Part model, mm, in its own coordinate system. Face numbers are marked on the shaded views. A direction names the side the tool comes from. Coordinates: 2 decimals unless noted, no trailing zeros. Loops run counter-clockwise (first coordinate to the right, second up) from the corner with the lowest first, then second, coordinate; pieces in that order, holes last. Notation, with made-up numbers: M 72,-26.5 L 88,-26.5 A19 cw 88,-9.5 Z; hole C -29,75.25 d3. An arc over 180 degrees is marked long. Use a Markdown table: item, result. Add a question column.
1) Band-saw the part on A-A (y = 19). State how many separate pieces and enclosed holes the cut face has, plus the area to 3 significant figures.
2) Wall check: probe 1 along Z at (x, y) = (1, 11.5); probe 2 along Z at (x, y) = (-2.5, 10.75); probe 3 along Y at (x, z) = (0, -39). Give the ranges that are in metal, low to high. Write a range as from..to.
3) Band-saw the part on D-D (z = -1.5). List the corners of the cut face in (x, y), plus the area to 3 significant figures.
4) Pull direction Z, two halves, no side cores. Call the marked faces 1, 2 and 3: released by +Z, released by -Z, zero draft, split by the parting line, or undercut.
5) Tool access for the marked faces 4 and 5: list every direction of +Z, -Z, +X, -X, +Y, -Y with a clear straight run to the whole face (end or side of a thin tool).
6) Band-saw the part on B-B (z = -31). List the corners of the cut face in (x, y), plus the area to 3 significant figures.
7) Pin check, flat tips, straight feed: pin 1 Ø4.5 at (y, z) = (7, 1) entering from +X; pin 2 Ø1.8 at (x, z) = (-13.5, 0.5) entering from +Y; pin 3 Ø3 at (x, y) = (0, 19) entering from +Z; pin 4 Ø3 at (x, z) = (0.5, -2.5) entering from +Y. Stop position of each tip, or through.
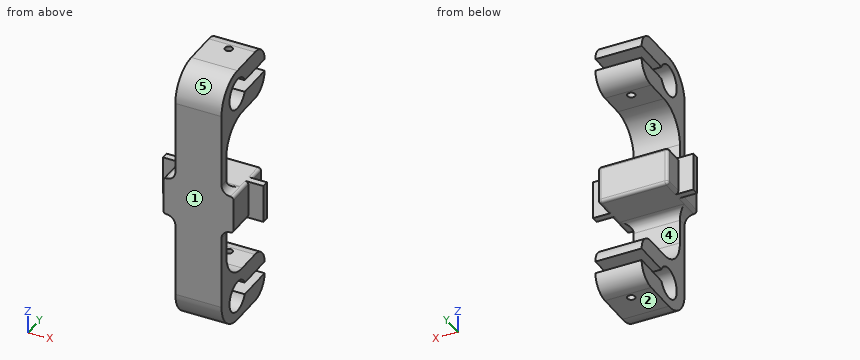
Autodesk Inventor part; units mm, degrees
ref_plane "YZ Plane" through (0, 0, 0) normal (1, 0, 0) x (0, 1, 0)
ref_plane "XZ Plane" through (0, 0, 0) normal (0, 1, 0) x (-1, 0, 0)
ref_plane "XY Plane" through (0, 0, 0) normal (0, 0, 1) x (1, 0, 0)
sketch "Schizzo1" plane through (0, 0, 0) normal (0, 1, 0) x (-1, 0, 0)
  line L0 (7.5, 43) -> (-7.5, 43)
  line L1 (-7.5, 43) -> (-7.5, -43)
  line L2 (-7.5, -43) -> (7.5, -43)
  line L3 (7.5, -43) -> (7.5, 43)
  line L4 (7.5, 43) -> (-7.5, -43) construction
  line L5 (-7.5, 43) -> (7.5, -43) construction
  point P0 (0, 0)
  dimension "d0" = 15
  dimension "d1" = 86
extrude "Estrusione1" add sketch "Schizzo1" along normal blind 3
sketch "Schizzo2" plane through (0, 3, 0) normal (0, 1, 0) x (1, 0, 0)
  line L0 (7.5, 43) -> (-7.5, 43)
  line L1 (-7.5, 43) -> (-7.5, 27)
  line L2 (-7.5, 27) -> (7.5, 27)
  line L3 (7.5, 27) -> (7.5, 43)
  line L4 (-7.5, 43) -> (-7.5, -43)
  line L5 (7.5, 43) -> (-7.5, 43)
  line L6 (-7.5, -43) -> (7.5, -43)
  line L7 (7.5, -43) -> (-7.5, -43)
  line L8 (-7.5, -43) -> (-7.5, -27)
  line L9 (-7.5, -27) -> (7.5, -27)
  line L10 (7.5, -27) -> (7.5, -43)
  point P0 (0, 0)
  dimension "d4" = 15
  dimension "d5" = 16
  dimension "d6" = 0
  dimension "d7" = 0
  dimension "d8" = 16
extrude "Estrusione2" add sketch "Schizzo2" along normal blind 24
sketch "Schizzo3" plane through (-7.5, 0, -43) normal (-1, 0, 0) x (0, 0, 1)
  line L0 (0, 0) -> (86, 0)
  line L1 (0, 0) -> (0, 27)
  line L2 (86, 0) -> (86, 27)
  circle A0 centre (8, 10) radius 5
  circle A1 centre (78, 10) radius 5
  point P0 (43, 0)
  dimension "d11" = 10
  dimension "d12" = 8
  dimension "d13" = 10
  dimension "d14" = 8
  dimension "d15" = 10
  dimension "d16" = 10
extrude "Estrusione3" cut sketch "Schizzo3" against normal blind 30
fillet "Raccordo1" radius 10 2 edges at (0, 3, -27) (0, 3, 27)
fillet "Raccordo2" radius 10 2 edges at (0, 0, -43) (0, 0, 43)
sketch "Schizzo4" plane through (0, 27, 0) normal (0, 1, 0) x (1, 0, 0)
  line L0 (7.5, 37) -> (-7.5, 37)
  line L1 (-7.5, 37) -> (-7.5, 33)
  line L2 (-7.5, 33) -> (7.5, 33)
  line L3 (7.5, 33) -> (7.5, 37)
  line L4 (7.5, 27) -> (7.5, 43)
  line L5 (7.5, 43) -> (-7.5, 43)
  line L6 (7.5, -33) -> (-7.5, -33)
  line L7 (-7.5, -33) -> (-7.5, -37)
  line L8 (-7.5, -37) -> (7.5, -37)
  line L9 (7.5, -37) -> (7.5, -33)
  line L10 (7.5, -43) -> (7.5, -27)
  line L11 (-7.5, -43) -> (7.5, -43)
  point P0 (0, 0)
  dimension "d21" = 15
  dimension "d22" = 4
  dimension "d23" = 0
  dimension "d24" = 6
  dimension "d25" = 15
  dimension "d26" = 4
  dimension "d27" = 0
  dimension "d28" = 6
extrude "Estrusione4" cut sketch "Schizzo4" against normal blind 15
sketch "Schizzo5" plane through (7.5, 27, -43) normal (0, 0, -1) x (-1, 0, 0)
  line L0 (0, 0) -> (15, 0)
  line L1 (15, -17) -> (15, 0)
  circle A0 centre (7.5, -8) radius 1.25
  point P0 (7.5, -27)
  dimension "d31" = 8
  dimension "d32" = 7.5
  dimension "d33" = 2.5
extrude "Estrusione5" cut sketch "Schizzo5" against normal blind 86
fillet "Raccordo3" radius 6 4 edges at (0, 27, 43) (0, 27, 27) (0, 27, -27) (0, 27, -43)
sketch "Schizzo6" plane through (0, 0, 0) normal (0, -1, 0) x (1, 0, 0)
  line L0 (-11.4, -6.2) -> (11.4, -6.2)
  line L1 (11.4, -6.2) -> (11.4, 6.2)
  line L2 (11.4, 6.2) -> (-11.4, 6.2)
  line L3 (-11.4, 6.2) -> (-11.4, -6.2)
  line L4 (-11.4, -6.2) -> (11.4, 6.2) construction
  line L5 (11.4, -6.2) -> (-11.4, 6.2) construction
  point P0 (0, 0)
  dimension "d37" = 22.8
  dimension "d38" = 12.4
extrude "Estrusione6" add sketch "Schizzo6" against normal blind 18
sketch "Schizzo7" plane through (11.4, 0, 6.2) normal (1, 0, 0) x (0, 0, -1)
  line L0 (0, 11.5) -> (12.4, 11.5)
  line L1 (12.4, 11.5) -> (12.4, 9.3)
  line L2 (12.4, 9.3) -> (0, 9.3)
  line L3 (0, 9.3) -> (0, 11.5)
  line L4 (0, 11.5) -> (12.4, 9.3) construction
  line L5 (12.4, 11.5) -> (0, 9.3) construction
  line L6 (12.4, 0) -> (0, 0)
  line L7 (12.4, 0) -> (12.4, 18)
  point P0 (6.2, 0)
  point P1 (6.2, 10.4)
  dimension "d41" = 12.4
  dimension "d42" = 2.2
  dimension "d43" = 9.3
  dimension "d44" = 0
extrude "Estrusione7" add sketch "Schizzo7" along normal blind 4.9
sketch "Schizzo8" plane through (-11.4, 0, -6.2) normal (-1, 0, 0) x (0, 0, 1)
  line L0 (0, 11.5) -> (12.4, 11.5)
  line L1 (12.4, 11.5) -> (12.4, 9.3)
  line L2 (12.4, 9.3) -> (0, 9.3)
  line L3 (0, 9.3) -> (0, 11.5)
  line L4 (0, 11.5) -> (12.4, 9.3) construction
  line L5 (12.4, 11.5) -> (0, 9.3) construction
  line L6 (12.4, 0) -> (0, 0)
  line L7 (12.4, 0) -> (12.4, 18)
  point P0 (6.2, 0)
  point P1 (6.2, 10.4)
  dimension "d47" = 12.4
  dimension "d48" = 2.2
  dimension "d49" = 9.3
  dimension "d50" = 0
extrude "Estrusione8" add sketch "Schizzo8" along normal blind 4.9
fillet "Raccordo4" radius 3 2 edges at (0, 3, 6.2) (0, 3, -6.2)
fillet "Raccordo5" radius 1 12 edges at (-11.4, 4.65, 6.2) (-11.4, 14.75, 6.2) (-11.4, 14.75, -6.2) (-11.4, 4.65, -6.2) (-11.4, 18, 0) (0, 18, -6.2) (0, 18, 6.2) (11.4, 4.65, -6.2) (11.4, 14.75, -6.2) (11.4, 18, 0) (11.4, 14.75, 6.2) (11.4, 4.65, 6.2)
fillet "Raccordo6" radius 2.9 8 edges at (-7.5, 4.5, -6.2) (-7.5, 1.5, -6.2) (-7.5, 1.5, 6.2) (-7.5, 4.5, 6.2) (7.5, 4.5, 6.2) (7.5, 1.5, 6.2) (7.5, 1.5, -6.2) (7.5, 4.5, -6.2)
properties part number "SupportGimbalAdafruit"
Entries:
| question | item | result |
|---|---|---|
| 1 | separate pieces | 8 |
| 1 | enclosed holes | 0 |
| 1 | area | 300 mm2 |
| 2 | probe 1 | -43..-39.77, -30.23..-26.89, -6.2..6.2, 26.89..30.23, 39.77..43 |
| 2 | probe 2 | -43..-39.94, -30.06..-26.74, -6.2..6.2, 26.74..30.06, 39.94..43 |
| 2 | probe 3 | 2..7, 13..17.75, 20.25..26.66 |
| 3 | outline | M -16.3,9.3 L -11.4,9.3 L -11.4,0 L 11.4,0 L 11.4,9.3 L 16.3,9.3 L 16.3,11.5 L 11.4,11.5 L 11.4,17 A1 ccw 10.4,18 L -10.4,18 A1 ccw -11.4,17 L -11.4,11.5 L -16.3,11.5 Z |
| 3 | area | 432 mm2 |
| 4 | face 1 | zero draft |
| 4 | face 2 | released by -Z |
| 4 | face 3 | undercut |
| 5 | face 4 | +X, -X, +Y |
| 5 | face 5 | +Z, +X, -X, -Y |
| 6 | outline | M -7.5,0 L 7.5,0 L 7.5,7 L -7.5,7 Z; M -7.5,13 L 7.5,13 L 7.5,26.66 L -7.5,26.66 Z; hole C 0,19 d2.5 |
| 6 | area | 305 mm2 |
| 7 | pin 1 | x = 11.4 |
| 7 | pin 2 | y = 11.5 |
| 7 | pin 3 | z = 43 |
| 7 | pin 4 | y = 18 |
